from build123d import *

# Parameters (mm, degrees)
SKETCH_1_W          = 20
SKETCH_1_H          = 17
EXTRUDE_1_DEPTH     = 3
SKETCH_4_W          = 17
SKETCH_4_H          = 20
EXTRUDE_2_DEPTH     = 3
EXTRUDE_3_DEPTH     = 2
EXTRUDE_4_DEPTH     = 2
CUT_EXTRUDE_2_DEPTH = 12
EXTRUDE_6_DEPTH     = 1
EXTRUDE_7_DEPTH     = 1


with BuildPart() as part:
    # 草图1 → 凸台-拉伸1 (new body)
    with BuildSketch(Plane(origin=(0, 0, 0), x_dir=(1, 0, 0), z_dir=(0, 1, 0))):
        with Locations((0.384615385, 1.297202797)):
            Rectangle(SKETCH_1_W, SKETCH_1_H)
        with BuildLine():
            Line((-2.115384615, 4.297202797), (2.884615385, 4.297202797))
            ThreePointArc((2.884615385, 4.297202797), (5.884615385, 1.297202797), (2.884615385, -1.702797203))
            Line((2.884615385, -1.702797203), (-2.115384615, -1.702797203))
            ThreePointArc((-2.115384615, -1.702797203), (-5.115384615, 1.297202797), (-2.115384615, 4.297202797))
        make_face(mode=Mode.SUBTRACT)
    extrude(amount=EXTRUDE_1_DEPTH)

    # 草图4 → 凸台-拉伸2 (add)
    with BuildSketch(Plane.ZY.offset(9.615384615)):
        with Locations((-1.297202797, 10)):
            Rectangle(SKETCH_4_W, SKETCH_4_H)
    extrude(amount=-EXTRUDE_2_DEPTH)

    # 草图6 → 凸台-拉伸3 (add)
    with BuildSketch(Plane.XY.offset(7.202797203)):
        Polygon((-6.615384615, 20), (10.384615385, 3), (-6.615384615, 3), align=None)
    extrude(amount=-EXTRUDE_3_DEPTH)

    # 草图7 → 凸台-拉伸4 (add)
    with BuildSketch(Plane(origin=(0, 0, -9.797202797), x_dir=(-1, 0, 0), z_dir=(0, 0, -1))):
        Polygon((6.615384615, 20), (6.615384615, 3), (-10.384615385, 3), align=None)
    extrude(amount=-EXTRUDE_4_DEPTH)

    # 草图5 → 切除-拉伸2 (cut)
    with BuildSketch(Plane(origin=(-6.615384615, 0, 0), x_dir=(0, 0, -1), z_dir=(1, 0, 0))):
        with BuildLine():
            Line((4.297202797, 12.5), (4.297202797, 7.5))
            ThreePointArc((4.297202797, 7.5), (1.297202797, 4.5), (-1.702797203, 7.5))
            Line((-1.702797203, 7.5), (-1.702797203, 12.5))
            ThreePointArc((-1.702797203, 12.5), (1.297202797, 15.5), (4.297202797, 12.5))
        make_face()
    extrude(amount=-CUT_EXTRUDE_2_DEPTH, mode=Mode.SUBTRACT)

    # 草图9 → 凸台-拉伸6 (add)
    with BuildSketch(Plane.ZY.offset(9.615384615)):
        with BuildLine():
            Line((-2.197202797, 18.65), (-0.397202797, 18.65))
            ThreePointArc((-0.397202797, 18.65), (0.502797203, 17.75), (-0.397202797, 16.85))
            Line((-0.397202797, 16.85), (-2.197202797, 16.85))
            ThreePointArc((-2.197202797, 16.85), (-3.097202797, 17.75), (-2.197202797, 18.65))
        make_face()
        with BuildLine():
            Line((-2.197202797, 3.15), (-0.397202797, 3.15))
            ThreePointArc((-0.397202797, 3.15), (0.502797203, 2.25), (-0.397202797, 1.35))
            Line((-0.397202797, 1.35), (-2.197202797, 1.35))
            ThreePointArc((-2.197202797, 1.35), (-3.097202797, 2.25), (-2.197202797, 3.15))
        make_face()
    extrude(amount=EXTRUDE_6_DEPTH)

    # 草图10 → 凸台-拉伸7 (add)
    with BuildSketch(Plane.XZ):
        with BuildLine():
            Line((-6.465384615, -0.397202797), (-6.465384615, -2.197202797))
            ThreePointArc((-6.465384615, -2.197202797), (-7.365384615, -3.097202797), (-8.265384615, -2.197202797))
            Line((-8.265384615, -2.197202797), (-8.265384615, -0.397202797))
            ThreePointArc((-8.265384615, -0.397202797), (-7.365384615, 0.502797203), (-6.465384615, -0.397202797))
        make_face()
        with BuildLine():
            Line((9.034615385, -0.397202797), (9.034615385, -2.197202797))
            ThreePointArc((9.034615385, -2.197202797), (8.134615385, -3.097202797), (7.234615385, -2.197202797))
            Line((7.234615385, -2.197202797), (7.234615385, -0.397202797))
            ThreePointArc((7.234615385, -0.397202797), (8.134615385, 0.502797203), (9.034615385, -0.397202797))
        make_face()
    extrude(amount=EXTRUDE_7_DEPTH)


solid = part.part
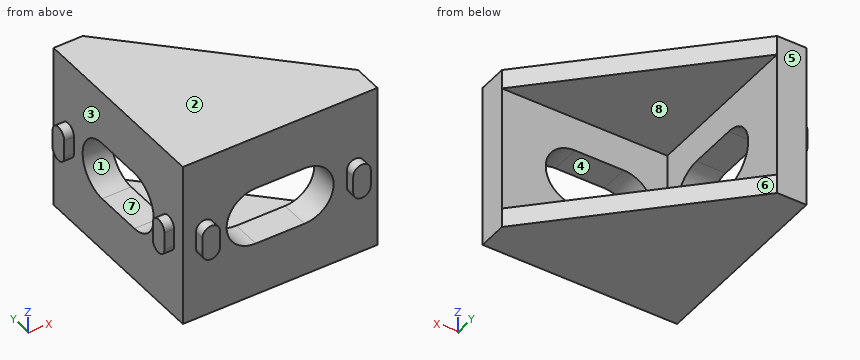
Can you work these out from the model? Positions are in its coordinate system, mm. Face numbers are marked on the shaded views. A direction names the side the tool comes from. Coordinates: 2 decimals unless noted, no trailing zeros. Order: outer loops, then holes, each group sorted by start corner. A loop starts at its lowest first (then second) coordinate and runs counter-clockwise, first axis right, second up. Notation, with made-up numbers: (16.25, -2) -> (61.25, -2) arc R9 ccw to (61.25, 3) -> close; hole circle Ø3 at (-18, 13). An arc over 180 degrees is marked (long way). Use one line per item in the form item = value.
Q1. Imagine slicing it at C-C, the plane y = 2.25. List the corners of the cut face in (x, z) for me.
From the geometry:
outline = (-10.62, -3.1) -> (-9.62, -3.1) -> (-9.62, -9.8) -> (10.38, -9.8) -> (10.38, 7.2) -> (-9.62, 7.2) -> (-9.62, 0.5) -> (-10.62, 0.5) -> close; hole (-2.12, -4.3) -> (2.88, -4.3) arc R3 ccw to (2.88, 1.7) -> (-2.12, 1.7) arc R3 ccw to start
Q2. Will these pins go through, and if not, where does the flat tip stop? P1, Ø1, axis at x = 3.5, z = -3, coming from the +Y side; P2, Ø1.1, axis at x = -10, z = -1, coming from the -Y side; P3, Ø4, axis at x = 5.5, z = 1, coming from the +Y side; P4, Ø0.5, axis at x = -10, z = -1, coming from the +Y side.
From the geometry:
P1 = through
P2 = 0
P3 = 3
P4 = 18.65
Q3. Which directions (+Z, -Z, +X, -X, +Y, -Y) give clear straight access to the entire face, cutting with the end or side of a thin tool? Please do the marked faces 4, 5, 6, 7 and 8.
From the geometry:
face_4 = +Y, -Y
face_5 = +Z, -Z, +X, -X, +Y
face_6 = +Z, -Z, +X, +Y
face_7 = +X, -X
face_8 = +X, +Y
Q4. We'd pull the mould along Z, two halves only. Please class the marked faces 1, 2 and 3: released by +Z, released by -Z, zero draft, split by the parting line, or undercut.
From the geometry:
face_1 = undercut
face_2 = released by +Z
face_3 = zero draft
Q5. Imagine slicing it at A-A, the plane y = 10.5. List the corners of the cut face in (x, z) for me, then the cut area to 3 significant figures.
From the geometry:
outline = (-9.62, -9.8) -> (2.88, -9.8) -> (2.88, -7.8) -> (-6.62, -7.8) -> (-6.62, -4.3) -> (-9.62, -4.3) -> close; (-9.62, 1.7) -> (-6.62, 1.7) -> (-6.62, 5.2) -> (2.88, 5.2) -> (2.88, 7.2) -> (-9.62, 7.2) -> close
area = 71.0 mm²
Q6. I need wall thicknesses on L1, parallel to Z at x = -2.25, y = 4.5; L2, parallel to Z at x = 0.25, y = 1.25; L3, parallel to Y at x = 7.25, z = -5.5. Which ranges of each line are inside material? Lowest first, please.
From the geometry:
L1 = -9.8 to -7.8, 5.2 to 7.2
L2 = -9.8 to -4.3, 1.7 to 7.2
L3 = 0 to 3
Q7. Imagine slicing it at B-B, the plane x = -9. List the corners of the cut face in (y, z) for me, then the cut area to 3 significant figures.
From the geometry:
outline = (0, -9.8) -> (20, -9.8) -> (20, 7.2) -> (0, 7.2) -> close; hole (7.5, -4.3) -> (12.5, -4.3) arc R3 ccw to (12.5, 1.7) -> (7.5, 1.7) arc R3 ccw to start
area = 282 mm²
Q8. Imagine slicing it at D-D, the plane x = 0. List the corners of the cut face in (y, z) for me.
From the geometry:
outline = (0, -9.8) -> (13.38, -9.8) -> (13.38, -7.8) -> (3, -7.8) -> (3, -4.3) -> (0, -4.3) -> close; (0, 1.7) -> (3, 1.7) -> (3, 5.2) -> (13.38, 5.2) -> (13.38, 7.2) -> (0, 7.2) -> close
